```python
from build123d import *

# Parameters (mm, degrees)
SKETCH1_R           = 2.5527
BOSS_EXTRUDE1_DEPTH = 3.175


with BuildPart() as part:
    # Sketch1 → Boss-Extrude1 (new body)
    with BuildSketch(Plane(origin=(0, 0, 0), x_dir=(1, 0, 0), z_dir=(0, 1, 0))):
        with BuildLine():
            Line((-75.4, 22.7), (-75.4, 0))
            Line((-75.4, 0), (-75.4, -22.7))
            ThreePointArc((-75.4, -22.7), (-73.935533906, -26.235533906), (-70.4, -27.7))
            Line((-70.4, -27.7), (70.4, -27.7))
            ThreePointArc((70.4, -27.7), (73.935533906, -26.235533906), (75.4, -22.7))
            Line((75.4, -22.7), (75.4, 0))
            Line((75.4, 0), (75.4, 22.7))
            ThreePointArc((75.4, 22.7), (73.935533906, 26.235533906), (70.4, 27.7))
            Line((70.4, 27.7), (-70.4, 27.7))
            ThreePointArc((-70.4, 27.7), (-73.935533906, 26.235533906), (-75.4, 22.7))
        make_face()
        with Locations(Location((-56.35, -21.35, 0), (0, 0, 270))):
            Circle(SKETCH1_R, mode=Mode.SUBTRACT)
        with Locations(Location((0, -21.35, 0), (0, 0, 270))):
            Circle(SKETCH1_R, mode=Mode.SUBTRACT)
        with Locations(Location((56.35, -21.35, 0), (0, 0, 270))):
            Circle(SKETCH1_R, mode=Mode.SUBTRACT)
        with Locations(Location((56.35, 21.35, 0), (0, 0, 270))):
            Circle(SKETCH1_R, mode=Mode.SUBTRACT)
        with Locations(Location((0, 21.35, 0), (0, 0, 270))):
            Circle(SKETCH1_R, mode=Mode.SUBTRACT)
        with Locations(Location((-56.35, 21.35, 0), (0, 0, 270))):
            Circle(SKETCH1_R, mode=Mode.SUBTRACT)
        with BuildLine():
            Line((45, 15), (-45, 15))
            ThreePointArc((-45, 15), (-48.535533906, 13.535533906), (-50, 10))
            Line((-50, 10), (-50, -10))
            ThreePointArc((-50, -10), (-48.535533906, -13.535533906), (-45, -15))
            Line((-45, -15), (45, -15))
            ThreePointArc((45, -15), (48.535533906, -13.535533906), (50, -10))
            Line((50, -10), (50, 10))
            ThreePointArc((50, 10), (48.535533906, 13.535533906), (45, 15))
        make_face(mode=Mode.SUBTRACT)
    extrude(amount=BOSS_EXTRUDE1_DEPTH)


solid = part.part
```
The model under review builds one solid part; all positions refer to its coordinate system, in mm. A direction names the side the tool comes from. Round coordinates to 2 decimals unless told otherwise and drop trailing zeros. Loops run counter-clockwise (first coordinate to the right, second up) from the corner with the lowest first, then second, coordinate; pieces in that order, holes last.
Item 1: For faces 1 (the face through (-1.06, 0, -18.85)), 2 (the face through (1, 2, -15)), list the 3-axis set-ups (+Z, -Z, +X, -X, +Y, -Y) from which the entire face can be reached by the end or side of a thin tool; tool diameter is ignored.
Determined:
face 1: +Z, -Z, +X, -X, -Y
face 2: +Y, -Y
Item 2: Take a section at C-C (y = 2.15). Write out the cut boundary in (x, z).
Determined:
outline: (-75.4, -22.7) arc R5 ccw to (-70.4, -27.7) - (70.4, -27.7) arc R5 ccw to (75.4, -22.7) - (75.4, 22.7) arc R5 ccw to (70.4, 27.7) - (-70.4, 27.7) arc R5 ccw to (-75.4, 22.7) - close; hole circle Ø5.11 at (-56.35, -21.35); hole circle Ø5.11 at (-56.35, 21.35); hole (-50, -10) arc R5 ccw to (-45, -15) - (45, -15) arc R5 ccw to (50, -10) - (50, 10) arc R5 ccw to (45, 15) - (-45, 15) arc R5 ccw to (-50, 10) - close; hole circle Ø5.11 at (0, -21.35); hole circle Ø5.11 at (0, 21.35); hole circle Ø5.11 at (56.35, -21.35); hole circle Ø5.11 at (56.35, 21.35)
Item 3: Mouldability with a two-part tool opening along X and no side actions: class faces 3 (the face through (-53.82, 1.57, 21.02)), 4 (the face through (-73.97, 1.57, 26.2)), 5 (the face through (-1, 2, 27.7)) as released by +X, released by -X, zero draft, split by the parting line, or undercut.
Determined:
face 3: undercut
face 4: released by -X
face 5: zero draft
Item 4: For line 1 (X direction, y = 2.1, z = 21.35); line 2 (Z direction, x = 37.5, y = 0.35); line 3 (X direction, y = 1.9, z = -9), list the stretches that pass through material, from the lowest coordinate up.
Determined:
line 1: x = -75.4 to -58.9, -53.8 to -2.55, 2.55 to 53.8, 58.9 to 75.4
line 2: z = -27.7 to -15, 15 to 27.7
line 3: x = -75.4 to -50, 50 to 75.4
Item 5: Clearance check with a flat-ended pin moving along its axis: pin 1 Ø4 at (x, z) = (56.35, -21.35) entering from -Y. State where the tip first meets the part, or that it passes through.
Determined:
pin 1: passes through
Item 6: Take a section at B-B (x = -35.5). Write out the cut boundary in (y, z) (3 decimals), then the cut area to 3 significant figures.
Determined:
outline: (0, -27.7) - (3.175, -27.7) - (3.175, -15) - (0, -15) - close; (0, 15) - (3.175, 15) - (3.175, 27.7) - (0, 27.7) - close
area: 80.6 mm2
Item 7: Take a section at D-D (x = 0). Write out the cut boundary in (y, z) (3 decimals).
Determined:
outline: (0, -27.7) - (3.175, -27.7) - (3.175, -23.903) - (0, -23.903) - close; (0, -18.797) - (3.175, -18.797) - (3.175, -15) - (0, -15) - close; (0, 15) - (3.175, 15) - (3.175, 18.797) - (0, 18.797) - close; (0, 23.903) - (3.175, 23.903) - (3.175, 27.7) - (0, 27.7) - close
Item 8: Take a section at A-A (z = -21.35). Write out the cut boundary in (x, y) (3 decimals), then the cut area to 3 significant figures.
Determined:
outline: (-75.4, 0) - (-58.903, 0) - (-58.903, 3.175) - (-75.4, 3.175) - close; (-53.797, 0) - (-2.553, 0) - (-2.553, 3.175) - (-53.797, 3.175) - close; (2.553, 0) - (53.797, 0) - (53.797, 3.175) - (2.553, 3.175) - close; (58.903, 0) - (75.4, 0) - (75.4, 3.175) - (58.903, 3.175) - close
area: 430 mm2
